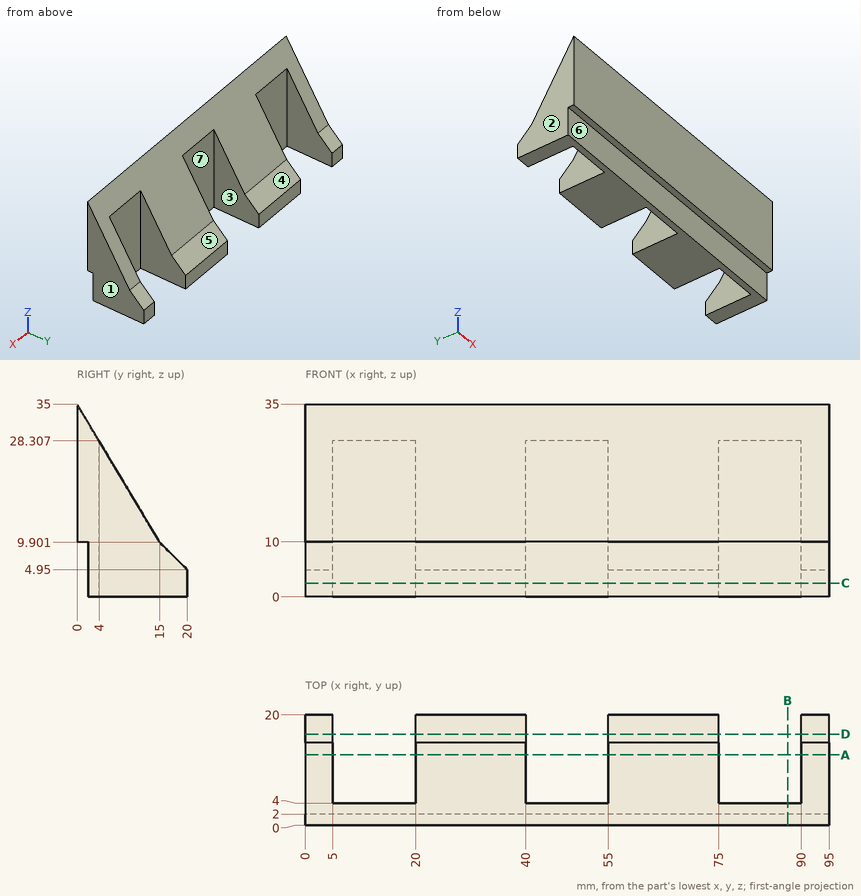
Answer from the drawing. Dimensions are ordinates in mm from the lowest x, y and z of the part. A direction names the side the tool comes from. Give positions to 0.01 mm unless a question says otherwise; leave off trailing zeros. Loops run counter-clockwise (first coordinate to the right, second up) from the corner with the lowest first, then second, coordinate; pieces in that order, holes last.
Item 1: For the marked faces 5, 6 and 7, determine the directions among +Z, -Z, +X, -X, +Y, -Y from which every point of the face is accessible in a straight line to the end or side of a thin tool.
Item 2: The part is cut by section A-A (y = 12.75). Write down the section's boundary in (x, z) (1 decimal).
Item 3: Each of these flat-tipped pins is pushed along its axis until it touches: pin 1 Ø3 at (x, z) = (38, 3) entering from -Y; pin 2 Ø7.5 at (x, z) = (44.5, 11) entering from +Y; pin 3 Ø8 at (x, y) = (65.5, 5.5) entering from +Z. Where does it stop, or does it pass through?
Item 4: The part is cut by section B-B (x = 87.5). Write down the section's boundary in (y, z), and give its area (3 significant figures).
Item 5: Find the intervals of material crossed by line 1 along X through (y, z) = (4.5, 10.5); line 2 along Y through (x, z) = (11.5, 11.5); line 3 along Y through (x, z) = (52, 2.5), in increasing order.
Item 6: The part is cut by section D-D (y = 16.5). Write down the section's boundary in (x, z) (1 decimal).
Item 7: The mould has two halves that part along X. Classify the marked faces 1, 2, 3 and 4: released by +X, released by -X, zero draft, split by the parting line, or undercut.
Item 8: The part is cut by section C-C (z = 2.5). Write down the section's boundary in (x, y).
Taken from the geometry:
1. face 5: +Z, +X, -X, +Y
1. face 6: -Z, +X, -X, -Y
1. face 7: +Z, -Z, +Y
2. outline: (0, 0) - (5, 0) - (5, 13.7) - (0, 13.7) - close; (20, 0) - (40, 0) - (40, 13.7) - (20, 13.7) - close; (55, 0) - (75, 0) - (75, 13.7) - (55, 13.7) - close; (90, 0) - (95, 0) - (95, 13.7) - (90, 13.7) - close
3. pin 1: stops at y = 2
3. pin 2: stops at y = 4
3. pin 3: stops at z = 32.49
4. outline: (0, 10) - (2, 10) - (2, 0) - (4, 0) - (4, 28.31) - (0, 35) - close
4. area: 107 mm2
5. line 1: x = 0 to 5, 20 to 40, 55 to 75, 90 to 95
5. line 2: y = 0 to 4
5. line 3: y = 2 to 4
6. outline: (0, 0) - (5, 0) - (5, 8.4) - (0, 8.4) - close; (20, 0) - (40, 0) - (40, 8.4) - (20, 8.4) - close; (55, 0) - (75, 0) - (75, 8.4) - (55, 8.4) - close; (90, 0) - (95, 0) - (95, 8.4) - (90, 8.4) - close
7. face 1: released by +X
7. face 2: released by -X
7. face 3: undercut
7. face 4: zero draft
8. outline: (0, 2) - (95, 2) - (95, 20) - (90, 20) - (90, 4) - (75, 4) - (75, 20) - (55, 20) - (55, 4) - (40, 4) - (40, 20) - (20, 20) - (20, 4) - (5, 4) - (5, 20) - (0, 20) - close
